Input: part model. Units: mm. Frame: model coordinates. A direction names the side the tool comes from. Coordinates: 2 decimals unless noted, no trailing zeros. Order: outer loops, then holes, each group sorted by start corner. A loop starts at its lowest first (then second) coordinate and runs counter-clockwise, first axis right, second up. Notation, with made-up numbers: (-22, 50.5) -> (16, 50.5) arc R33 cw to (16, 86.5) -> close; hole circle Ø7 at (40, -24.5). An arc over 180 degrees is marked (long way). Answer as CSV lines item,"result".
from build123d import *

# Parameters (mm, degrees)
BOSS_EXTRUDE1_DEPTH = 20
SKETCH2_W           = 5
SKETCH2_H           = 27.5
CUT_EXTRUDE2_DEPTH  = 5
SKETCH3_W           = 5
SKETCH3_H           = 27.5
CUT_EXTRUDE3_DEPTH  = 5
BOSS_EXTRUDE2_DEPTH = 15
SKETCH5_W           = 30
SKETCH5_H           = 2.5
BOSS_EXTRUDE3_DEPTH = 10
SKETCH6_W           = 15
SKETCH6_H           = 5
CUT_EXTRUDE4_DEPTH  = 25
SKETCH7_R           = 10
BOSS_EXTRUDE4_DEPTH = 10
SKETCH8_R           = 5
CUT_EXTRUDE5_DEPTH  = 310
BOSS_EXTRUDE5_DEPTH = 10
SKETCH11_R          = 2.5
CUT_EXTRUDE6_DEPTH  = 300


with BuildPart() as part:
    # Sketch1 → Boss-Extrude1 (new body)
    with BuildSketch(Plane.XY):
        Polygon((-80, 0), (-65, 10), (-65, 15), (-55, 15), (-55, 10), (-25, 10), (-25, 15), (-15, 15), (-15, 10), (0, 0), (0, -20), (-15, -30), (-15, -35), (-25, -35), (-25, -30), (-55, -30), (-55, -35), (-65, -35), (-65, -30), (-80, -20), align=None)
    extrude(amount=BOSS_EXTRUDE1_DEPTH)

    # Sketch2 → Cut-Extrude2 (cut)
    with BuildSketch(Plane.ZY.offset(80)):
        with Locations((2.5, -10)):
            Rectangle(SKETCH2_W, SKETCH2_H)
    extrude(amount=-CUT_EXTRUDE2_DEPTH, mode=Mode.SUBTRACT)

    # Sketch3 → Cut-Extrude3 (cut)
    with BuildSketch(Plane(origin=(0, 0, 0), x_dir=(0, 0, -1), z_dir=(1, 0, 0))):
        with Locations((-2.5, -10)):
            Rectangle(SKETCH3_W, SKETCH3_H)
    extrude(amount=-CUT_EXTRUDE3_DEPTH, mode=Mode.SUBTRACT)

    # Sketch4 → Boss-Extrude2 (add)
    with BuildSketch(Plane.XY.offset(20)):
        with BuildLine():
            Line((-55, 10), (-25, 10))
            ThreePointArc((-25, 10), (-5, -10), (-25, -30))
            Line((-25, -30), (-55, -30))
            ThreePointArc((-55, -30), (-75, -10), (-55, 10))
        make_face()
    extrude(amount=BOSS_EXTRUDE2_DEPTH)

    # Sketch5 → Boss-Extrude3 (add)
    with BuildSketch(Plane(origin=(0, 0, 0), x_dir=(-1, 0, 0), z_dir=(0, 0, -1))):
        with Locations((40, -31.25)):
            Rectangle(SKETCH5_W, SKETCH5_H)
        with Locations((40, 11.25)):
            Rectangle(SKETCH5_W, SKETCH5_H)
    extrude(amount=-BOSS_EXTRUDE3_DEPTH)

    # Sketch6 → Cut-Extrude4 (cut)
    with BuildSketch(Plane.XY.offset(35)):
        with Locations((-40, -27.5)):
            Rectangle(SKETCH6_W, SKETCH6_H)
        with Locations((-40, 7.5)):
            Rectangle(SKETCH6_W, SKETCH6_H)
    extrude(amount=-CUT_EXTRUDE4_DEPTH, mode=Mode.SUBTRACT)

    # Sketch7 → Boss-Extrude4 (add)
    with BuildSketch(Plane.XY.offset(35)):
        with Locations((-40, -10)):
            Circle(SKETCH7_R)
    extrude(amount=BOSS_EXTRUDE4_DEPTH)

    # Sketch8 → Cut-Extrude5 (cut)
    with BuildSketch(Plane.XY.offset(45)):
        with Locations((-40, -10)):
            Circle(SKETCH8_R)
    extrude(amount=-CUT_EXTRUDE5_DEPTH, mode=Mode.SUBTRACT)

    # Sketch10 → Boss-Extrude5 (add)
    with BuildSketch(Plane.XY.offset(35)):
        with BuildLine():
            Line((-73.540496218, -17.5), (-66.040496218, -17.5))
            ThreePointArc((-66.040496218, -17.5), (-58.540496218, -10), (-66.040496218, -2.5))
            Line((-66.040496218, -2.5), (-73.540496218, -2.5))
            ThreePointArc((-73.540496218, -2.5), (-75, -10), (-73.540496218, -17.5))
        make_face()
        with BuildLine():
            Line((-6.459503782, -17.5), (-13.959503782, -17.5))
            ThreePointArc((-13.959503782, -17.5), (-21.459503782, -10), (-13.959503782, -2.5))
            Line((-13.959503782, -2.5), (-6.459503782, -2.5))
            ThreePointArc((-6.459503782, -2.5), (-5, -10), (-6.459503782, -17.5))
        make_face()
    extrude(amount=BOSS_EXTRUDE5_DEPTH)

    # Sketch11 → Cut-Extrude6 (cut)
    with BuildSketch(Plane.XY.offset(45)):
        with Locations((-66.040496218, -10)):
            Circle(SKETCH11_R)
        with Locations((-13.959503782, -10)):
            Circle(SKETCH11_R)
    extrude(amount=-CUT_EXTRUDE6_DEPTH, mode=Mode.SUBTRACT)


solid = part.part
1. Contact query for flat-ended pins moving along their axis: pin 1 (2.5 mm diameter, centred on y = -32.5, z = 11.5, fed in from +X); pin 2 (2 mm diameter, centred on x = -70, z = 40.5, fed in from +Y); pin 3 (1 mm diameter, centred on y = -18.5, z = 35, fed in from +X). Output: stop coordinate, or through.
Findings:
pin 1,"stops at x = -15"
pin 2,"stops at y = -2.5"
pin 3,"stops at x = -6.67"
2. Cut plane A-A (z = 16). State how many separate pieces and enclosed holes the cut face has, plus the area to 3 significant figures.
Findings:
separate pieces,"1"
enclosed holes,"3"
area,"2,830 mm2"
3. Reachability of faces 1 (the face through (-76, -12, 20)), 2 (the face through (-4, -12, 20)), 3 (the face through (-50, -10, 40)), 4 (the face through (-47.5, -28, 23)), 5 (the face through (-51, 10, 22)) from +Z, -Z, +X, -X, +Y, -Y: full face, straight path, thin tool, end or side. Return the list, or none.
Findings:
face 1,"+Z, -X"
face 2,"+Z, +X"
face 3,"+Z"
face 4,"+Z, -Y"
face 5,"+Z, +Y"
4. Ray query, line 1 along X through (y, z) = (-9, 4); line 2 along X through (y, z) = (-9, 9); line 3 along Z through (x, y) = (-24.5, -15). Return the intervals inside material, ascending.
Findings:
line 1,"x = -75 to -68.33, -63.75 to -44.9, -35.1 to -16.25, -11.67 to -5"
line 2,"x = -80 to -68.33, -63.75 to -44.9, -35.1 to -16.25, -11.67 to 0"
line 3,"z = 0 to 35"
5. Cut plane D-D (y = 2). Return the cut outline in (x, z), plus the area to 3 significant figures.
Findings:
outline,"(-77, 5) -> (-75, 5) -> (-75, 0) -> (-5, 0) -> (-5, 5) -> (-3, 5) -> (-3, 20) -> (-9, 20) -> (-9, 35) -> (-71, 35) -> (-71, 20) -> (-77, 20) -> close"
area,"2,390 mm2"
6. Mould query, pull axis X, two halves, no side actions, for faces 6 (the face through (-7.605, 5.07, 9.86)), 7 (the face through (-32.5, -28, 23)), 8 (the face through (-10, -2.5, 40)). Classes: released by +X, released by -X, zero draft, split by the parting line, or undercut.
Findings:
face 6,"released by +X"
face 7,"undercut"
face 8,"zero draft"
7. Cut plane B-B (x = -40). Return the cut outline in (y, z).
Findings:
outline,"(-32.5, 0) -> (-15, 0) -> (-15, 45) -> (-20, 45) -> (-20, 35) -> (-25, 35) -> (-25, 10) -> (-32.5, 10) -> close; (-5, 0) -> (12.5, 0) -> (12.5, 10) -> (5, 10) -> (5, 35) -> (0, 35) -> (0, 45) -> (-5, 45) -> close"
